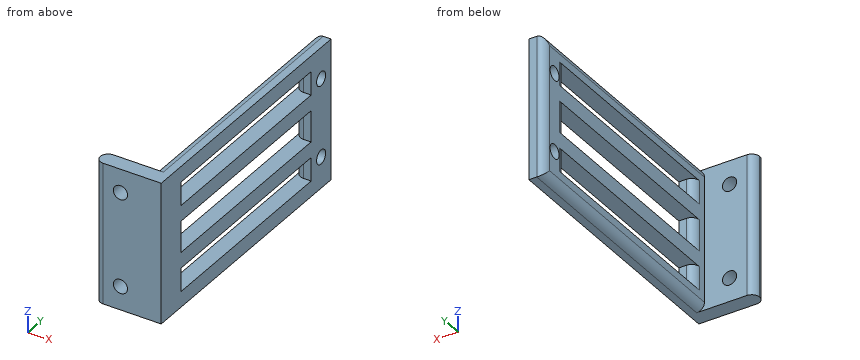
from build123d import *

# Parameters (mm, degrees)
F0_W     = 16
F0_H     = 5
F1_DEPTH = 45
F2_R     = 2.25
F3_DEPTH = 5
F4_W     = 65
F4_H     = 7.5
F4_R     = 2.25
F4_H_2   = 10
F5_DEPTH = 5
F6_R     = 2.49999


# Not quite as in the source:
# - a fillet or chamfer is up to 0.001 mm smaller than in the source, because OpenCascade refuses the exact size
# - a feature names something its author has since deleted; it is built from what else it names


with BuildPart() as f1:
    # F0 (on Top) → F1 (new body)
    with BuildSketch(Plane.XY):
        Polygon((-4.1043104958, 55.0339419188), (-4.1043104958, -24.9660580812), (-4.1043104958, -29.9660580812), (0.8956895042, -29.9660580812), (0.8956895042, 55.0339419188), align=None)
        with Locations((-12.1043104958, -27.4660580812)):
            Rectangle(F0_W, F0_H)
    extrude(amount=F1_DEPTH)

    # F2 (on face) → F3 (cut, through all)
    with BuildSketch(Plane(origin=(0, -24.9660580812, 0), x_dir=(-1, 0, 0), z_dir=(0, 1, 0))):
        with Locations((12.1043104958, 7.5)):
            Circle(F2_R)
        with Locations((12.1043104958, 37.5)):
            Circle(F2_R)
    extrude(amount=-F3_DEPTH, mode=Mode.SUBTRACT)

    # F4 (on face) → F5 (cut, through all)
    with BuildSketch(Plane(origin=(-4.1043104958, 0, 0), x_dir=(0, -1, 0), z_dir=(-1, 0, 0))):
        with Locations((-12.5339419188, 8.75)):
            Rectangle(F4_W, F4_H)
        with Locations((-50.0339419188, 35)):
            Circle(F4_R)
        with Locations((-50.0339419188, 10)):
            Circle(F4_R)
        with Locations((-12.5339419188, 22.5)):
            Rectangle(F4_W, F4_H_2)
        with Locations((-12.5339419188, 36.25)):
            Rectangle(F4_W, F4_H)
    extrude(amount=-F5_DEPTH, mode=Mode.SUBTRACT)

    # F6 (radius 2.5 in the source; OpenCascade refuses exactly that, so slightly less here)
    f6_edges = [f1.edges().sort_by_distance(p)[0] for p in [
        (-4.10431, 15.033942, 0),
        (-4.10431, 55.033942, 22.5),
        (-4.10431, 15.033942, 45),
        (-4.10431, 45.033942, 8.75),
        (-4.10431, 45.033942, 22.5),
        (-4.10431, 45.033942, 36.25),
        (-4.10431, -19.966058, 8.75),
        (-4.10431, -19.966058, 22.5),
        (-4.10431, -19.966058, 36.25),
        (-20.10431, -24.966058, 22.5),
        (-20.10431, -29.966058, 22.5),
    ]]
    fillet(f6_edges, radius=F6_R)


solid = f1.part
The listing builds one solid part. Answer for the finished solid, in the listing's coordinates (mm). Round coordinates to 2 decimals unless told otherwise and drop trailing zeros. Loops run counter-clockwise (first coordinate to the right, second up) from the corner with the lowest first, then second, coordinate; pieces in that order, holes last. Notation, with made-up numbers: M 76,-32 L 109,-32 A16 ccw 109,-12 Z; hole C 3.25,74 d8. An arc over 180 degrees is marked long. Write each question's results on one line, items separated by ' | '. Start each with the question number.
1) Straight lines are drawn through the part: probe 1 along Z at (x, y) = (-0.75, -5); probe 2 along Z at (x, y) = (-1.75, 48); probe 3 along Y at (x, z) = (-0.25, 26.5). For each, find the intervals that lie inside material, in ascending order.
2) Find section B-B on y = 34.5. Write down the section's boundary in (x, z).
3) Find section C-C on x = -12.25. Write down the section's boundary in (y, z), plus the area to 3 significant figures.
4) Each of these flat-tipped pins is pushed along its axis until it touches: pin 1 (4 mm diameter, centred on x = -10.5, z = 14, fed in from +Y); pin 2 (4 mm diameter, centred on y = 15, z = 5.5, fed in from -X). Where does it stop, or does it pass through?
Final values:
1) probe 1: 0 to 5, 12.5 to 17.5, 27.5 to 32.5, 40 to 45 | probe 2: 0 to 9.04, 10.96 to 34.04, 35.96 to 45 | probe 3: -29.97 to -19.97, 45.03 to 55.03
2) outline: M -4.1,2.5 A2.5 ccw -1.6,0 L 0.9,0 L 0.9,5 L -4.1,5 Z; M -4.1,12.5 L 0.9,12.5 L 0.9,17.5 L -4.1,17.5 Z; M -4.1,27.5 L 0.9,27.5 L 0.9,32.5 L -4.1,32.5 Z; M -4.1,40 L 0.9,40 L 0.9,45 L -1.6,45 A2.5 ccw -4.1,42.5 Z
3) outline: M -29.97,0 L -24.97,0 L -24.97,5.25 L -29.97,5.25 Z; M -29.97,9.75 L -24.97,9.75 L -24.97,35.25 L -29.97,35.25 Z; M -29.97,39.75 L -24.97,39.75 L -24.97,45 L -29.97,45 Z | area: 180 mm²
4) pin 1: y = -24.97 | pin 2: x = -4.1
